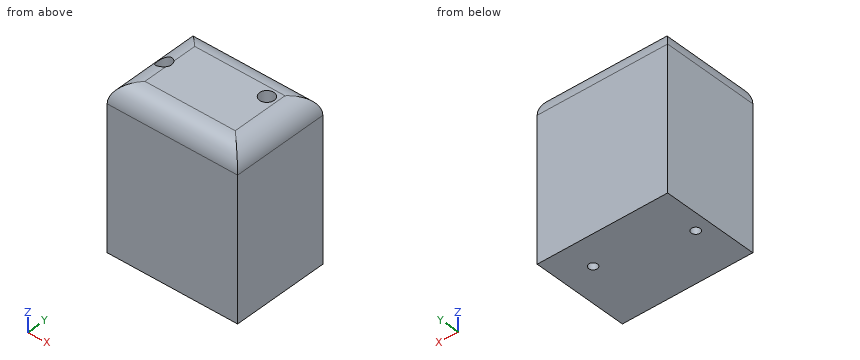
from build123d import *

# Parameters (mm, degrees)
SKIZZE1_W                                           = 135.069444444
SKIZZE1_H                                           = 100
AUFSATZ_LINEAR_AUSTRAGEN1_DEPTH                     = 168
SCHNITT_LINEAR_AUSTRAGEN1_DEPTH                     = 222.286589794
SCHNITT_LINEAR_AUSTRAGEN2_DEPTH                     = 207.845204696
SPIEGELN2_COPY_1_DEPTH                              = 222.286589794
SPIEGELN2_COPY_2_DEPTH                              = 222.286589794
STIRNSENKUNG_F_R_M8_SENKSCHRAUBE_KOPF_B_D           = 9
STIRNSENKUNG_F_R_M8_SENKSCHRAUBE_KOPF_B_CBORE_D     = 15
STIRNSENKUNG_F_R_M8_SENKSCHRAUBE_KOPF_B_CBORE_DEPTH = 161
STIRNSENKUNG_F_R_M8_SENKSCHRAUBE_KO_2_D             = 9
STIRNSENKUNG_F_R_M8_SENKSCHRAUBE_KO_2_CBORE_D       = 15
STIRNSENKUNG_F_R_M8_SENKSCHRAUBE_KO_2_CBORE_DEPTH   = 161


with BuildPart() as part:
    # Skizze1 → Aufsatz-Linear austragen1 (new body)
    with BuildSketch(Plane.XY):
        Rectangle(SKIZZE1_W, SKIZZE1_H)
    extrude(amount=AUFSATZ_LINEAR_AUSTRAGEN1_DEPTH)

    # Skizze2 → Schnitt-Linear austragen1 (cut, through all)
    with BuildSketch(Plane(origin=(67.534722222, 0, 0), x_dir=(0, 0, -1), z_dir=(1, 0, 0))):
        with BuildLine():
            Line((-147.230769231, 50), (18.556111772, 50))
            Line((18.556111772, 50), (-294.033910821, 102.758784569))
            Line((-294.033910821, 102.758784569), (-168, -33.660289563))
            Line((-168, -33.660289563), (-168, 29.230769231))
            ThreePointArc((-168, 29.230769231), (-161.916833148, 43.916833148), (-147.230769231, 50))
        make_face()
    schnitt_linear_austragen1 = extrude(amount=-SCHNITT_LINEAR_AUSTRAGEN1_DEPTH, mode=Mode.SUBTRACT)

    # Skizze3 → Schnitt-Linear austragen2 (cut, through all)
    with BuildSketch(Plane.XZ.offset(50)):
        with BuildLine():
            Line((67.534722222, 147.230769231), (67.534722222, 12.080316404))
            Line((67.534722222, 12.080316404), (116.298873036, 236.387140366))
            Line((116.298873036, 236.387140366), (-16.125567341, 168))
            Line((-16.125567341, 168), (46.765491453, 168))
            ThreePointArc((46.765491453, 168), (61.45155537, 161.916833148), (67.534722222, 147.230769231))
        make_face()
    schnitt_linear_austragen2 = extrude(amount=-SCHNITT_LINEAR_AUSTRAGEN2_DEPTH, mode=Mode.SUBTRACT)

    # Spiegeln1: Schnitt-Linear austragen1 across plane
    add(schnitt_linear_austragen1.mirror(Plane.ZX), mode=Mode.SUBTRACT)

    # Spiegeln2: Schnitt-Linear austragen2 across plane
    add(schnitt_linear_austragen2.mirror(Plane(origin=(0, 0, 0), x_dir=(0, 0, 1), z_dir=(1, 0, 0))), mode=Mode.SUBTRACT)

    # Spiegeln2 copy 1 sketch → Spiegeln2 copy 1 (cut, through all)
    with BuildSketch(Plane(origin=(-67.534722222, 0, 0), x_dir=(0, 0, -1), z_dir=(-1, 0, 0))):
        with BuildLine():
            Line((-147.230769231, 50), (18.556111772, 50))
            Line((18.556111772, 50), (-294.033910821, 102.758784569))
            Line((-294.033910821, 102.758784569), (-168, -33.660289563))
            Line((-168, -33.660289563), (-168, 29.230769231))
            ThreePointArc((-168, 29.230769231), (-161.916833148, 43.916833148), (-147.230769231, 50))
        make_face()
    extrude(amount=-SPIEGELN2_COPY_1_DEPTH, mode=Mode.SUBTRACT)

    # Spiegeln2 copy 2 sketch → Spiegeln2 copy 2 (cut, through all)
    with BuildSketch(Plane(origin=(-67.534722222, 0, 0), x_dir=(0, 0, -1), z_dir=(-1, 0, 0))):
        with BuildLine():
            Line((-147.230769231, -50), (18.556111772, -50))
            Line((18.556111772, -50), (-294.033910821, -102.758784569))
            Line((-294.033910821, -102.758784569), (-168, 33.660289563))
            Line((-168, 33.660289563), (-168, -29.230769231))
            ThreePointArc((-168, -29.230769231), (-161.916833148, -43.916833148), (-147.230769231, -50))
        make_face()
    extrude(amount=-SPIEGELN2_COPY_2_DEPTH, mode=Mode.SUBTRACT)

    # Stirnsenkung f_r M8 Senkschraube _Kopf B (through all)
    with Locations(Plane.XY.offset(168)):
        with Locations((-52.534722222, 0)):
            CounterBoreHole(STIRNSENKUNG_F_R_M8_SENKSCHRAUBE_KOPF_B_D / 2, STIRNSENKUNG_F_R_M8_SENKSCHRAUBE_KOPF_B_CBORE_D / 2, STIRNSENKUNG_F_R_M8_SENKSCHRAUBE_KOPF_B_CBORE_DEPTH)

    # Stirnsenkung f_r M8 Senkschraube _Ko 2 (through all)
    with Locations(Plane.XY.offset(168)):
        with Locations((36.765491453, 19.230769231)):
            CounterBoreHole(STIRNSENKUNG_F_R_M8_SENKSCHRAUBE_KO_2_D / 2, STIRNSENKUNG_F_R_M8_SENKSCHRAUBE_KO_2_CBORE_D / 2, STIRNSENKUNG_F_R_M8_SENKSCHRAUBE_KO_2_CBORE_DEPTH)


solid = part.part
The model under review builds one solid part; all positions refer to its coordinate system, in mm. Coordinates: 2 decimals unless noted, no trailing zeros. Write each loop counter-clockwise with the first axis right and the second up, starting at its lowest first coordinate (ties: lowest second). Pieces come first, ordered by that corner, then holes. Notation, with made-up numbers: (39.5, 41.5) -> (96.5, 41.5) arc R14 cw to (96.5, 46.5) -> close; hole circle Ø9 at (68, 45.25). An arc over 180 degrees is marked (long way). Answer in a Markdown table with one row per item.
1. Wall thickness on probe 1 along Y at (x, z) = (38, 121); probe 2 along Y at (x, z) = (-53, 19); probe 3 along Z at (x, y) = (-31, -30.5): over which ranges is each line inside the solid? List them lowest first. Write a range as [from, to].
Answers below:
| item | result |
|---|---|
| probe 1 | y = [-50, 11.83], [26.63, 50] |
| probe 2 | y = [-50, -7.49], [7.49, 50] |
| probe 3 | z = [0, 167.96] |
2. Clearance check with a flat-ended pin moving along its axis: pin 1 Ø14.5 at (x, y) = (-52.53, 0) entering from +Z. State where the tip first meets the part, or that it passes through.
Answers below:
| item | result |
|---|---|
| pin 1 | stops at z = 7 |
3. We need section B-B, the plane z = 19. State the section outline as (x, y) points.
Answers below:
| item | result |
|---|---|
| outline | (-67.53, -50) -> (67.53, -50) -> (67.53, 50) -> (-67.53, 50) -> close; hole circle Ø15 at (-52.53, 0); hole circle Ø15 at (36.77, 19.23) |
4. We need section A-A, the plane y = 0. State the section outline as (x, z) points.
Answers below:
| item | result |
|---|---|
| outline | (-67.53, 0) -> (-57.03, 0) -> (-57.03, 7) -> (-60.03, 7) -> (-60.03, 163.21) arc R20.77 ccw to (-67.53, 147.23) -> close; (-48.03, 0) -> (67.53, 0) -> (67.53, 147.23) arc R20.77 ccw to (46.77, 168) -> (-45.03, 168) -> (-45.03, 7) -> (-48.03, 7) -> close |
